from build123d import *

# Parameters (mm, degrees)
SKETCH1_W                 = 45.5
SKETCH1_H                 = 67.5
BOSS_EXTRUDE1_DEPTH       = 1.25
SKETCH21_W                = 1.925
SKETCH21_H                = 1
BOSS_EXTRUDE10_DEPTH      = 8
SKETCH7_W                 = 45.5
SKETCH7_H                 = 67.5
SKETCH7_W_2               = 41.5
SKETCH7_H_2               = 63.5
BOSS_EXTRUDE4_DEPTH       = 22
SKETCH18_W                = 13
SKETCH18_H                = 8
CUT_EXTRUDE10_DEPTH       = 2
BOSS_EXTRUDE20_DEPTH      = 4
SKETCH49_R                = 1.75
BOSS_EXTRUDE21_DEPTH      = 35
SKETCH50_W                = 13.462095761
SKETCH50_H                = 5
SKETCH50_W_2              = 20.764616991
SKETCH50_H_2              = 20
CUT_EXTRUDE12_DEPTH       = 12
FILLET7_R                 = 1
M4_CLEARANCE_HOLE1_D      = 4.8
SKETCH42_W                = 7.3
SKETCH42_H                = 7.3
SKETCH42_W_2              = 19.24
SKETCH42_H_2              = 2
SKETCH42_W_3              = 7.65
SKETCH42_H_3              = 7.65
BOSS_EXTRUDE19_DEPTH      = 8
F_3_0MM_DOWEL_HOLE1_D     = 3.1
F_3_0MM_DOWEL_HOLE1_DEPTH = 2.8
F_3_0MM_DOWEL_HOLE1_TIP   = 0.931333959
SKETCH52_W                = 10
SKETCH52_H                = 6
CUT_EXTRUDE13_DEPTH       = 12
FILLET11_R                = 1.5
FILLET13_R                = 1
FILLET15_R                = 1
FILLET14_R                = 1
SKETCH53_R                = 7
CUT_EXTRUDE14_DEPTH       = 0.75
SKETCH54_W                = 2.5
SKETCH54_H                = 62
BOSS_EXTRUDE22_DEPTH      = 3


with BuildPart() as part:
    # Sketch1 → Boss-Extrude1 (new body)
    with BuildSketch(Plane.XY):
        Rectangle(SKETCH1_W, SKETCH1_H)
    extrude(amount=BOSS_EXTRUDE1_DEPTH)

    # Sketch21 → Boss-Extrude10 (add)
    with BuildSketch(Plane.XY.offset(1.25)):
        with Locations((-19.7875, 30.75)):
            Rectangle(SKETCH21_W, SKETCH21_H)
        with Locations((-3.8125, 30.75)):
            Rectangle(SKETCH21_W, SKETCH21_H)
    extrude(amount=BOSS_EXTRUDE10_DEPTH)

    # Sketch7 → Boss-Extrude4 (add)
    with BuildSketch(Plane.XY.offset(1.25)):
        Rectangle(SKETCH7_W, SKETCH7_H)
        Rectangle(SKETCH7_W_2, SKETCH7_H_2, mode=Mode.SUBTRACT)
    extrude(amount=BOSS_EXTRUDE4_DEPTH)

    # Sketch18 → Cut-Extrude10 (cut)
    with BuildSketch(Plane(origin=(0, 33.75, 0), x_dir=(1, 0, 0), z_dir=(0, 1, 0))):
        with Locations((-12.425, -6.15)):
            Rectangle(SKETCH18_W, SKETCH18_H)
    extrude(amount=-CUT_EXTRUDE10_DEPTH, mode=Mode.SUBTRACT)

    # Sketch48 → Boss-Extrude20 (add)
    with BuildSketch(Plane.XY.offset(23.25)):
        Polygon((22.75, 33.75), (32.75, 33.75), (32.75, 12.75), (22.75, 12.75), (22.75, 15.75), (28.75, 15.75), (28.75, 30.75), (22.75, 30.75), align=None)
        Polygon((-22.75, 30.75), (-28.75, 30.75), (-28.75, 15.75), (-22.75, 15.75), (-22.75, 12.75), (-32.75, 12.75), (-32.75, 33.75), (-22.75, 33.75), align=None)
    extrude(amount=-BOSS_EXTRUDE20_DEPTH)

    # Sketch49 → Boss-Extrude21 (add)
    with BuildSketch(Plane.XZ.offset(33.75)):
        with BuildLine():
            Line((27.75, 20.25), (22.75, 20.25))
            Line((22.75, 20.25), (22.75, 23.25))
            Line((22.75, 23.25), (24.75, 23.25))
            ThreePointArc((24.75, 23.25), (29.871320344, 25.371320344), (27.75, 20.25))
        make_face()
        with Locations(Location((27.75, 23.25, 0), (0, 0, 270))):
            Circle(SKETCH49_R, mode=Mode.SUBTRACT)
    extrude(amount=-BOSS_EXTRUDE21_DEPTH)

    # Sketch50 → Cut-Extrude12 (cut)
    with BuildSketch(Plane(origin=(22.75, 0, 0), x_dir=(0, 0, -1), z_dir=(1, 0, 0))):
        with Locations((-22.765361812, -31.25)):
            Rectangle(SKETCH50_W, SKETCH50_H)
        with Locations((-19.114101197, -13.75)):
            Rectangle(SKETCH50_W_2, SKETCH50_H_2)
    extrude(amount=CUT_EXTRUDE12_DEPTH, mode=Mode.SUBTRACT)

    # Fillet7
    fillet7_edges = [part.edges().sort_by_distance(p)[0] for p in [
        (-18.925, 32.75, 2.15),
        (-18.925, 32.75, 10.15),
        (-5.925, 32.75, 10.15),
        (-5.925, 32.75, 2.15),
    ]]
    fillet(fillet7_edges, radius=FILLET7_R)

    # M4 Clearance Hole1 (through all)
    with Locations(Plane.XY.offset(1.25)):
        with Locations((-12, 24.25), (8, 24.25), (8, -10.75), (-12, -10.75)):
            Hole(M4_CLEARANCE_HOLE1_D / 2)

    # Sketch42 → Boss-Extrude19 (add)
    with BuildSketch(Plane.XY.offset(1.25)):
        with Locations((0.8, 24.1)):
            Rectangle(SKETCH42_W, SKETCH42_H)
        with Locations((16.04, 24.1)):
            Rectangle(SKETCH42_W, SKETCH42_H)
        with Locations((8.42, 15.806169598)):
            Rectangle(SKETCH42_W_2, SKETCH42_H_2)
        with Locations((0.975, -22.925)):
            Rectangle(SKETCH42_W_3, SKETCH42_H_3)
        with Locations((13.675, -22.925)):
            Rectangle(SKETCH42_W_3, SKETCH42_H_3)
        with Locations((13.675, -2.605)):
            Rectangle(SKETCH42_W_3, SKETCH42_H_3)
        with Locations((0.975, -2.605)):
            Rectangle(SKETCH42_W_3, SKETCH42_H_3)
    extrude(amount=BOSS_EXTRUDE19_DEPTH)

    # Ø3.0mm Dowel Hole1
    with Locations(Plane.XY.offset(9.25)):
        with Locations((0.8, 24.1), (16.04, 24.1), (13.675, -2.605), (0.975, -2.605), (0.975, -22.925), (13.675, -22.925)):
            Hole(F_3_0MM_DOWEL_HOLE1_D / 2, depth=F_3_0MM_DOWEL_HOLE1_DEPTH)
            with Locations((0, 0, -(F_3_0MM_DOWEL_HOLE1_DEPTH + F_3_0MM_DOWEL_HOLE1_TIP / 2))):  # 118° drill point
                Cone(0, F_3_0MM_DOWEL_HOLE1_D / 2, F_3_0MM_DOWEL_HOLE1_TIP, mode=Mode.SUBTRACT)

    # Sketch52 → Cut-Extrude13 (cut)
    with BuildSketch(Plane(origin=(0, 31.75, 0), x_dir=(-1, 0, 0), z_dir=(0, -1, 0))):
        with Locations((-7.73, -13.25)):
            Rectangle(SKETCH52_W, SKETCH52_H)
    extrude(amount=-CUT_EXTRUDE13_DEPTH, mode=Mode.SUBTRACT)

    # Fillet11
    fillet11_edges = [part.edges().sort_by_distance(p)[0] for p in [
        (2.73, 32.75, 10.25),
        (2.73, 32.75, 16.25),
        (12.73, 32.75, 16.25),
        (12.73, 32.75, 10.25),
    ]]
    fillet(fillet11_edges, radius=FILLET11_R)

    # Fillet13
    fillet13_edges = [part.edges().sort_by_distance(p)[0] for p in [
        (22.75, -33.75, 11.625),
        (0, 33.75, 0),
        (22.75, 0, 0),
        (0, -33.75, 0),
        (-22.75, 0, 0),
        (-22.75, -33.75, 11.625),
        (-22.75, 33.75, 9.625),
        (22.75, 33.75, 9.625),
    ]]
    fillet(fillet13_edges, radius=FILLET13_R)

    # Fillet15
    fillet15_edges = [part.edges().sort_by_distance(p)[0] for p in [
        (25.75, 30.75, 23.25),
        (28.75, 23.25, 23.25),
        (32.75, 23.25, 23.25),
        (25.75, 15.75, 23.25),
        (27.75, 12.75, 23.25),
        (32.75, 12.75, 21.25),
        (32.75, 33.75, 21.25),
        (27.25, 33.75, 19.25),
        (25.75, 30.75, 19.25),
        (28.75, 23.25, 19.25),
        (32.75, 23.25, 19.25),
        (27.75, 12.75, 19.25),
        (25.75, 15.75, 19.25),
        (0, 33.75, 23.25),
    ]]
    fillet(fillet15_edges, radius=FILLET15_R)

    # Fillet14
    fillet14_edges = [part.edges().sort_by_distance(p)[0] for p in [
        (-25.75, 30.75, 19.25),
        (-28.75, 23.25, 19.25),
        (-25.75, 15.75, 19.25),
        (-27.75, 12.75, 19.25),
        (-32.75, 23.25, 19.25),
        (-32.75, 12.75, 21.25),
        (-27.25, 33.75, 19.25),
        (-32.75, 33.75, 20.75),
        (-27.75, 12.75, 23.25),
        (-28.75, 23.25, 23.25),
        (-25.75, 30.75, 23.25),
        (-32.75, 22.75, 23.25),
        (-32.75, 33.457106781, 22.957106781),
    ]]
    fillet(fillet14_edges, radius=FILLET14_R)

    # Sketch53 → Cut-Extrude14 (cut)
    with BuildSketch(Plane.ZY.offset(22.75)):
        with Locations((23.25, -12.898378645)):
            Circle(SKETCH53_R)
    extrude(amount=-CUT_EXTRUDE14_DEPTH, mode=Mode.SUBTRACT)

    # Sketch54 → Boss-Extrude22 (add)
    with BuildSketch(Plane.XY.offset(1.25)):
        with Locations((-19.5, -0.75)):
            Rectangle(SKETCH54_W, SKETCH54_H)
        with Locations((-4.1, -0.75)):
            Rectangle(SKETCH54_W, SKETCH54_H)
    extrude(amount=BOSS_EXTRUDE22_DEPTH)


solid = part.part
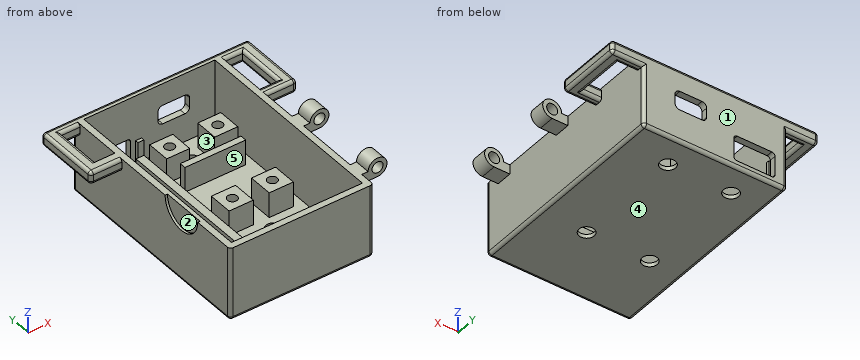
Verification items for the finished model (mm, model axes). Face numbers are marked on the shaded views. A direction names the side the tool comes from. Give positions to 0.01 mm unless a question says otherwise; leave off trailing zeros. Order: outer loops, then holes, each group sorted by start corner. A loop starts at its lowest first (then second) coordinate and runs counter-clockwise, first axis right, second up. Notation, with made-up numbers: (36, 4.25) -> (87, 4.25) arc R15 ccw to (87, 20.25) -> close; hole circle Ø10 at (-21, 57.25). An arc over 180 degrees is marked (long way). Answer as CSV lines item,"result".
Q1. Sectioned sample at C-C on x = -12. Record the cut outline in (y, z).
Solutions:
outline,"(-33.75, 1) arc R1 ccw to (-32.75, 0) -> (-13.15, 0) -> (-13.15, 1.25) -> (-31.75, 1.25) -> (-31.75, 23.25) -> (-33.75, 23.25) -> close; (-8.35, 0) -> (21.85, 0) -> (21.85, 1.25) -> (-8.35, 1.25) -> close; (26.65, 0) -> (32.75, 0) arc R1 ccw to (33.75, 1) -> (33.75, 2.15) -> (31.75, 2.15) -> (31.75, 1.25) -> (26.65, 1.25) -> close; (31.75, 10.15) -> (33.75, 10.15) -> (33.75, 22.25) arc R1 ccw to (32.75, 23.25) -> (31.75, 23.25) -> close"
Q2. Scan lines: probe 1 along Y at (x, z) = (19, 7.25); probe 2 along X at (y, z) = (21.5, 5.25); probe 3 along X at (y, z) = (28.5, 22). Record each from-to range of solid material in increasing order.
Solutions:
probe 1,"y = -33.75 to -31.75, 20.45 to 27.75, 31.75 to 33.75"
probe 2,"x = -22.75 to -20.75, -2.85 to 4.45, 12.39 to 19.69, 20.75 to 22.75"
probe 3,"x = -32.75 to -28.75, -22.75 to -20.75, 20.75 to 22.75, 28.75 to 32.75"
Q3. Sectioned sample at A-A on y = 4. Record the cut outline in (x, z), plus the area to 3 significant figures.
Solutions:
outline,"(-22.75, 1) arc R1 ccw to (-21.75, 0) -> (21.75, 0) arc R1 ccw to (22.75, 1) -> (22.75, 23.25) -> (20.75, 23.25) -> (20.75, 1.25) -> (-2.85, 1.25) -> (-2.85, 4.25) -> (-5.35, 4.25) -> (-5.35, 1.25) -> (-18.25, 1.25) -> (-18.25, 4.25) -> (-20.75, 4.25) -> (-20.75, 23.25) -> (-22.75, 23.25) -> close"
area,"159 mm²"
Q4. Release check for a two-part mould opening along X. For the marked faces 1, 2 and 3 record: +X half, -X half, draft (parallel to the pull), parting line (faces both ways), or undercut.
Solutions:
face 1,"draft"
face 2,"-X half"
face 3,"undercut"
Q5. Depth check by flat-ended pin: pin 1 (2 mm diameter, centred on y = 20.5, z = 9.5, fed in from +X); pin 2 (1 mm diameter, centred on x = -22.5, z = 17.5, fed in from -Y); pin 3 (4 mm diameter, centred on y = -1, z = 7, fed in from -X); pin 4 (4.5 mm diameter, centred on x = 8, y = -10.75, fed in from +Z). Enter the tip coordinate at first touch or a pass-through.
Solutions:
pin 1,"stops at x = 22.75"
pin 2,"stops at y = -33.72"
pin 3,"stops at x = -22.75"
pin 4,"passes through"
Q6. Sectioned sample at B-B on x = 8. Record the cut outline in (y, z), plus the area to 3 significant figures.
Solutions:
outline,"(-33.75, 1) arc R1 ccw to (-32.75, 0) -> (-13.15, 0) -> (-13.15, 1.25) -> (-31.75, 1.25) -> (-31.75, 23.25) -> (-33.75, 23.25) -> close; (-8.35, 0) -> (21.85, 0) -> (21.85, 1.25) -> (16.81, 1.25) -> (16.81, 9.25) -> (14.81, 9.25) -> (14.81, 1.25) -> (-8.35, 1.25) -> close; (26.65, 0) -> (32.75, 0) arc R1 ccw to (33.75, 1) -> (33.75, 10.25) -> (31.75, 10.25) -> (31.75, 1.25) -> (26.65, 1.25) -> close; (31.75, 16.25) -> (33.75, 16.25) -> (33.75, 22.25) arc R1 ccw to (32.75, 23.25) -> (31.75, 23.25) -> close"
area,"164 mm²"
Q7. Access from +Z, -Z, +X, -X, +Y, -Y to the whole of each face (thin tool, end or side, straight path). Record for the marked faces 4 and 5.
Solutions:
face 4,"-Z, +X, -X, +Y, -Y"
face 5,"+Z"
